The listing builds one solid part. Answer for the finished solid, in the listing's coordinates (mm). Give positions to 0.01 mm unless a question says otherwise; leave off trailing zeros. Loops run counter-clockwise (first coordinate to the right, second up) from the corner with the lowest first, then second, coordinate; pieces in that order, holes last. Notation, with made-up numbers: (-21, 57.5) - (-10, 57.5) arc R7 cw to (-10, 66.5) - close; hole circle Ø3 at (15.25, -27.5). An arc over 180 degrees is marked (long way). Write each question's results on one line, items separated by ' | '.
from build123d import *

# Parameters (mm, degrees)
SKETCH_1_W      = 2.7
SKETCH_1_H      = 20.3
SKETCH_1_R      = 0.4
SKETCH_1_W_2    = 4
SKETCH_1_H_2    = 3
EXTRUDE_1_DEPTH = 1


with BuildPart() as part:
    # Sketch 1 → Extrude 1 (new body)
    # profile 1 of 3: a face of its own
    with BuildSketch(Plane(origin=(0, 0, 0), x_dir=(1, 0, 0), z_dir=(0, 1, 0))):
        with Locations((1.35, -10.15)):
            Rectangle(SKETCH_1_W, SKETCH_1_H)
        with Locations(Location((1.2, -17.15, 0), (0, 0, 270))):
            Circle(SKETCH_1_R, mode=Mode.SUBTRACT)
        with Locations(Location((1.2, -3.15, 0), (0, 0, 270))):
            Circle(SKETCH_1_R, mode=Mode.SUBTRACT)
    # profile 2 of 3: a face of its own
    with BuildSketch(Plane(origin=(0, 0, 0), x_dir=(1, 0, 0), z_dir=(0, 1, 0))):
        with Locations((4.7, -14.3)):
            Rectangle(SKETCH_1_W_2, SKETCH_1_H_2)
    # profile 3 of 3: a face of its own
    with BuildSketch(Plane(origin=(0, 0, 0), x_dir=(1, 0, 0), z_dir=(0, 1, 0))):
        with Locations((4.7, -6)):
            Rectangle(SKETCH_1_W_2, SKETCH_1_H_2)
    extrude(amount=EXTRUDE_1_DEPTH)


solid = part.part
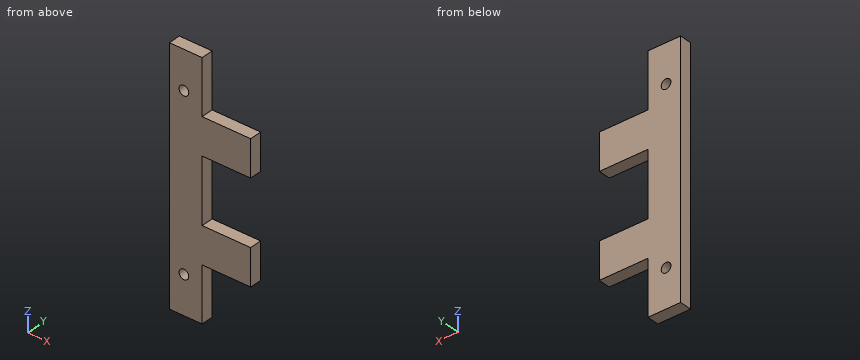
Item 1: A cutting plane is placed at B-B, the plane y = 0.6. Determine the outline of the cut face in (x, z), plus the area to 3 significant figures.
Values found:
outline: (0, 0) - (2.7, 0) - (2.7, 4.5) - (6.7, 4.5) - (6.7, 7.5) - (2.7, 7.5) - (2.7, 12.8) - (6.7, 12.8) - (6.7, 15.8) - (2.7, 15.8) - (2.7, 20.3) - (0, 20.3) - close; hole circle Ø0.8 at (1.2, 3.15); hole circle Ø0.8 at (1.2, 17.15) | area: 77.8 mm²
Item 2: Find the intervals of material crossed by line 1 along Z through (x, y) = (1.5, 0.6); line 2 along X through (y, z) = (0.4, 3.15); line 3 along Z through (x, y) = (4, 0.45), in increasing order. Write a range as [from, to].
Values found:
line 1: z = [0, 2.89], [3.41, 16.89], [17.41, 20.3] | line 2: x = [0, 0.8], [1.6, 2.7] | line 3: z = [4.5, 7.5], [12.8, 15.8]
Item 3: A cutting plane is placed at C-C, the plane z = 17.15. Determine the outline of the cut face in (x, y).
Values found:
outline: (0, 0) - (0.8, 0) - (0.8, 1) - (0, 1) - close; (1.6, 0) - (2.7, 0) - (2.7, 1) - (1.6, 1) - close
Item 4: A cutting plane is placed at D-D, the plane x = 5.5. Determine the outline of the cut face in (y, z), plus the area to 3 significant figures.
Values found:
outline: (0, 4.5) - (1, 4.5) - (1, 7.5) - (0, 7.5) - close; (0, 12.8) - (1, 12.8) - (1, 15.8) - (0, 15.8) - close | area: 6.00 mm²
Item 5: A cutting plane is placed at A-A, the plane x = 1.2. Determine the outline of the cut face in (y, z).
Values found:
outline: (0, 0) - (1, 0) - (1, 2.75) - (0, 2.75) - close; (0, 3.55) - (1, 3.55) - (1, 16.75) - (0, 16.75) - close; (0, 17.55) - (1, 17.55) - (1, 20.3) - (0, 20.3) - close
Item 6: Flat-ended cylindrical pins translate along their axes: P1, Ø3, axis at x = 3.5, z = 12, coming from the -Y side; P2, Ø0.5, axis at y = 0.5, z = 10.5, coming from the +X side. Find the tip coordinate at first contact, or state that the pin passes through.
Values found:
P1: stops at y = 0 | P2: stops at x = 2.7
